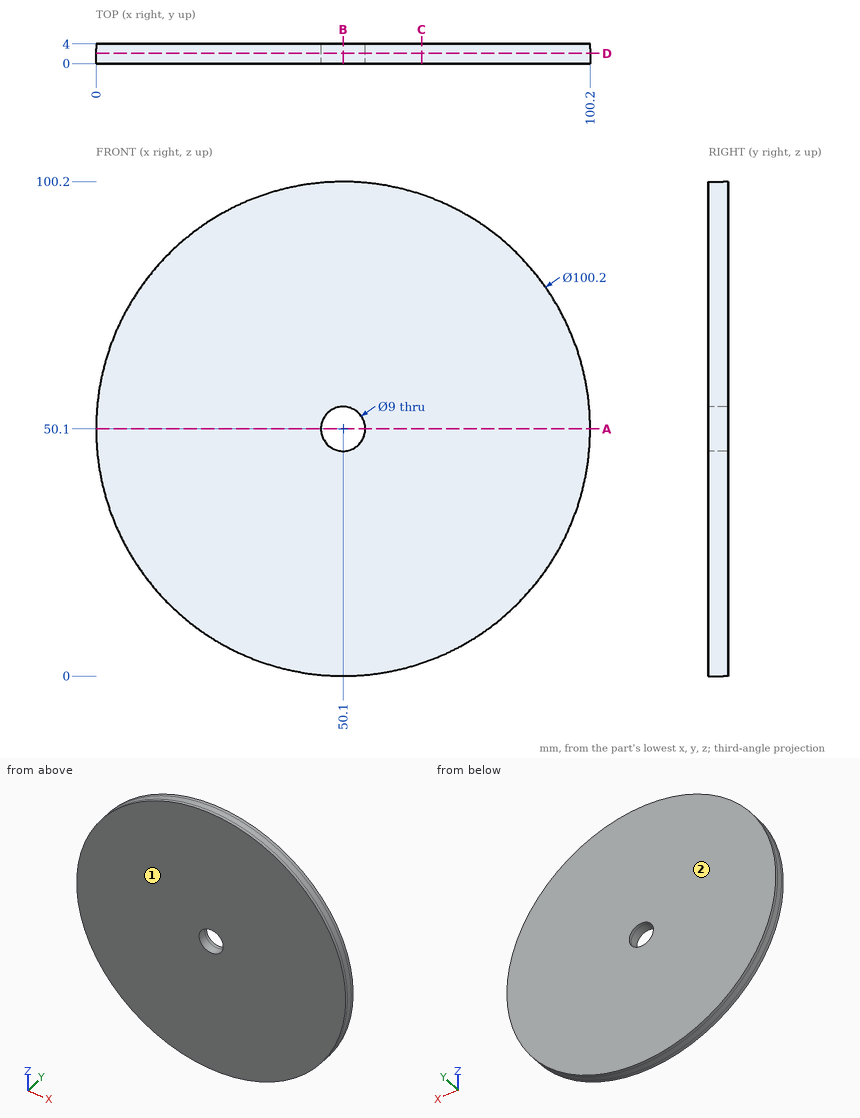
Source: three-view drawing plus pictorial views. Frame: mm from the lowest corner of the part. Round coordinates to 2 decimals unless told otherwise and drop trailing zeros. Loops run counter-clockwise (first coordinate to the right, second up) from the corner with the lowest first, then second, coordinate; pieces in that order, holes last.
1. Ray query, L1, parallel to Z at x = 50.1, y = 3.65; L2, parallel to Z at x = 68.5, y = 2.1; L3, parallel to X at y = 1.1, z = 20. Return the intervals inside material, ascending.
2. Contact query for flat-ended pins moving along their axis: pin 1 (8 mm diameter, centred on x = 50.1, z = 50.1, fed in from -Y); pin 2 (1.5 mm diameter, centred on y = 0.5, z = 34, fed in from +X). Output: stop coordinate, or through.
3. Section query A-A on z = 50.1. Output: boundary loops of the cut face in (x, y).
4. Section query C-C on x = 66. Output: boundary loops of the cut face in (y, z), and give its area (3 significant figures).
5. Section query D-D on y = 2.1. Output: boundary loops of the cut face in (x, z).
6. Section query B-B on x = 50.1. Output: boundary loops of the cut face in (y, z).
7. Mould query, pull axis Y, two halves, no side actions, for the marked faces 1 and 2. Classes: released by +Y, released by -Y, zero draft, split by the parting line, or undercut.
Answers below:
1. L1: z = 0 to 45.6, 54.6 to 100.2
1. L2: z = 3.5 to 96.7
1. L3: x = 10.05 to 90.15
2. pin 1: passes through
2. pin 2: stops at x = 97.79
3. outline: (0, 0) - (45.6, 0) - (45.6, 4) - (0, 4) - close; (54.6, 0) - (100.2, 0) - (100.2, 4) - (54.6, 4) - close
4. outline: (0, 2.59) - (4, 2.59) - (4, 97.61) - (0, 97.61) - close
4. area: 380 mm2
5. outline: circle Ø100.2 at (50.1, 50.1); hole circle Ø9 at (50.1, 50.1)
6. outline: (0, 0) - (4, 0) - (4, 45.6) - (0, 45.6) - close; (0, 54.6) - (4, 54.6) - (4, 100.2) - (0, 100.2) - close
7. face 1: released by -Y
7. face 2: released by +Y
